Can you work these out from the model? Positions are in its coordinate system, mm. Face numbers are marked on the shaded views. A direction names the side the tool comes from. Give positions to 0.01 mm unless a question says otherwise; leave off trailing zeros. Loops run counter-clockwise (first coordinate to the right, second up) from the corner with the lowest first, then second, coordinate; pieces in that order, holes last. Notation, with made-up numbers: (36, -10.5) -> (79, -10.5) arc R23 ccw to (79, 11.5) -> close; hole circle Ø11 at (-10, -31.5). An arc over 180 degrees is marked (long way). One line per question, with ' | ' between items.
Autodesk Inventor part; units mm, degrees
ref_plane "YZ Plane" through (0, 0, 0) normal (1, 0, 0) x (0, 1, 0)
ref_plane "XZ Plane" through (0, 0, 0) normal (0, 1, 0) x (-1, 0, 0)
ref_plane "XY Plane" through (0, 0, 0) normal (0, 0, 1) x (1, 0, 0)
ref_plane "Work Plane1" through (0, 0, 0) normal (0, 0, 1) x (1, 0, 0)
ref_plane "Work Plane2" through (0, 0, 0) normal (0, 0, 1) x (1, 0, 0)
ref_plane "Work Plane3" through (0, 0, 0) normal (0, 0, 1) x (1, 0, 0)
sketch "Sketch1" plane through (0, 0, 0) normal (0, 0, 1) x (1, 0, 0)
  line L0 (232.95, -21.7) -> (142.052, -21.7)
  line L1 (142.052, -21.7) -> (142.052, 21.7)
  line L2 (142.052, 21.7) -> (232.95, 21.7)
  line L3 (232.95, 21.7) -> (232.95, -21.7)
  line L4 (148.402, -7.551111) -> (148.402, 7.551111)
  line L5 (226.6, 7.551111) -> (226.6, -7.551111)
  line L6 (205.085111, -9) -> (189.982889, -9)
  line L7 (188.534, 9) -> (206.534, 9)
  circle A0 centre (217.6, 0) radius 2.775
  circle A1 centre (217.6, 0) radius 5.315
  circle A2 centre (197.534, 0) radius 5.315
  circle A3 centre (177.468, 0) radius 5.315
  circle A4 centre (157.402, 0) radius 5.315
  circle A5 centre (217.6, 0) radius 2.775
  circle A6 centre (197.534, 0) radius 2.775
  circle A7 centre (177.468, 0) radius 2.775
  circle A8 centre (157.402, 0) radius 2.775
  line L8 (208.075, 9.906) -> (227.125, 9.906)
  line L9 (227.125, 9.906) -> (227.125, -9.906)
  line L10 (227.125, -9.906) -> (208.075, -9.906)
  line L11 (208.075, -9.906) -> (208.075, 9.906)
  line L12 (208.075, 9.906) -> (227.125, -9.906) construction
  line L13 (227.125, 9.906) -> (208.075, -9.906) construction
  line L14 (207.059, -9.906) -> (188.009, -9.906)
  line L15 (207.059, 9.906) -> (207.059, -9.906)
  line L16 (188.009, 9.906) -> (207.059, 9.906)
  line L17 (188.009, -9.906) -> (188.009, 9.906)
  line L18 (186.993, -9.906) -> (167.943, -9.906)
  line L19 (186.993, 9.906) -> (186.993, -9.906)
  line L20 (167.943, 9.906) -> (186.993, 9.906)
  line L21 (167.943, -9.906) -> (167.943, 9.906)
  line L22 (166.927, -9.906) -> (147.877, -9.906)
  line L23 (166.927, 9.906) -> (166.927, -9.906)
  line L24 (147.877, 9.906) -> (166.927, 9.906)
  line L25 (147.877, -9.906) -> (147.877, 9.906)
  point P0 (0, 0)
  dimension "d0" = 6.35
  dimension "d1" = 6.35
  dimension "d3" = 12.7
  dimension "d4" = 12.7
  dimension "d5" = 2.54
  dimension "d8" = 20.066
  dimension "d15" = 20.066
  dimension "d20" = 19.05
  dimension "d21" = 19.812
  dimension "d24" = 20.066
extrude "Extrusion1" add sketch "Sketch1" along normal blind 5 contours A1
sketch "Sketch3" plane through (0, 0, 0) normal (0, 0, 1) x (1, 0, 0)
  line L0 (225.6, -8) -> (209.6, -8)
  line L1 (225.6, 8) -> (225.6, -8)
  line L2 (209.6, 8) -> (225.6, 8)
  line L3 (209.6, -8) -> (209.6, 8)
  line L4 (210.616, -6.984) -> (224.584, -6.984)
  line L5 (224.584, -6.984) -> (224.584, 6.984)
  line L6 (224.584, 6.984) -> (210.616, 6.984)
  line L7 (210.616, 6.984) -> (210.616, -6.984)
  circle A0 centre (217.6, 0) radius 5.315
  circle A1 centre (217.6, 0) radius 2.775
  point P0 (0, 0)
  dimension "d40" = 1.016
sketch "Sketch3 outline for Extrusion3" plane through (0, 0, 0) normal (0, 0, 1) x (1, 0, 0)
  line L0 (210.616, -6.984) -> (224.584, -6.984)
  line L1 (210.616, 6.984) -> (210.616, -6.984)
  line L2 (224.584, -6.984) -> (224.584, 6.984)
  line L3 (224.584, 6.984) -> (210.616, 6.984)
  circle A0 centre (217.6, 0) radius 2.775
extrude "Extrusion3" add sketch "Sketch3 outline for Extrusion3" along normal blind 4 draft -15
pattern_linear "Rectangular Pattern1" count 4 spacing 20.066 along (-1, 0, 0) of "Extrusion3", "Extrusion1"
ref_plane "Work Plane4" through (0, 0, 0) normal (0, 0, 1) x (1, 0, 0)
sketch "Sketch4" plane through (0, 0, 0) normal (0, 0, 1) x (1, 0, 0)
  line L0 (-228.6, 12.7) -> (228.6, 12.7)
  line L1 (228.6, -12.7) -> (-228.6, -12.7)
  line L2 (228.6, 12.7) -> (228.6, -12.7)
  line L3 (146.336, 9) -> (146.336, -9)
  line L4 (228.6, 12.7) -> (146.336, 12.7)
  line L5 (146.336, 12.7) -> (146.336, -12.7)
  line L6 (146.336, -12.7) -> (228.6, -12.7)
  line L7 (228.6, -12.7) -> (228.6, 12.7)
  point P0 (0, 0)
extrude "Extrusion4" add sketch "Sketch4" against normal blind 4
properties part number "Bottom Holder"
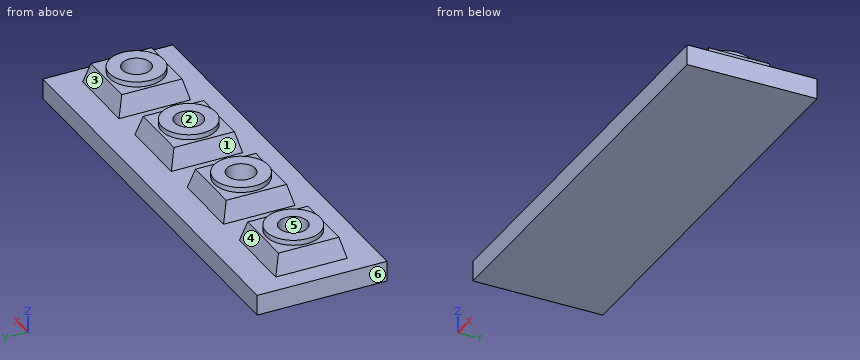
Q1. If we section it at A-A (x = 217.6): Write out the boundary of the cut face in (y, z) (3 decimals), plus the area to 3 significant figures.
Entries:
outline: (-12.7, -4) -> (12.7, -4) -> (12.7, 0) -> (6.984, 0) -> (5.912, 4) -> (5.315, 4) -> (5.315, 5) -> (2.775, 5) -> (2.775, 0) -> (-2.775, 0) -> (-2.775, 5) -> (-5.315, 5) -> (-5.315, 4) -> (-5.912, 4) -> (-6.984, 0) -> (-12.7, 0) -> close | area: 136 mm²
Q2. If I drill on probe 1 along Z at (x, y) = (215.5, 0.25); probe 2 along Y at (x, z) = (217.6, 2.7) (3 decimals); probe 3 along Y at (x, z) = (175.5, 1.5), over which ranges is the centre line in solid material (lowest first)? Write a range as from..to.
Entries:
probe 1: -4..0 | probe 2: -6.261..-2.775, 2.775..6.261 | probe 3: -6.58..-1.96, 1.96..6.58
Q3. If we section it at D-D (x = 168.5): Write out the boundary of the cut face in (y, z).
Entries:
outline: (-12.7, -4) -> (12.7, -4) -> (12.7, 0) -> (-12.7, 0) -> close
Q4. If we section it at B-B (x = 181): Write out the boundary of the cut face in (y, z), plus the area to 3 significant figures.
Entries:
outline: (-12.7, -4) -> (12.7, -4) -> (12.7, 0) -> (6.98, 0) -> (5.91, 4) -> (3.97, 4) -> (3.97, 5) -> (-3.97, 5) -> (-3.97, 4) -> (-5.91, 4) -> (-6.98, 0) -> (-12.7, 0) -> close | area: 161 mm²
Q5. For pin 1 Ø6 at (x, y) = (176, 1.5) entering from +Z; pin 2 Ø1.7 at (x, y) = (198, 0.5) entering from +Z; pin 3 Ø2 at (y, z) = (5.5, 2.5) entering from +X; pin 4 Ø1.5 at (x, z) = (158, 1) entering from -Y, each with a flat end and sliding along its axis, tell me the tip position at first contact or that it passes through.
Entries:
pin 1: z = 5 | pin 2: z = 0 | pin 3: x = 224.18 | pin 4: y = -6.92
Q6. If we section it at C-C (x = 156.5): Write out the boundary of the cut face in (y, z).
Entries:
outline: (-12.7, -4) -> (12.7, -4) -> (12.7, 0) -> (6.98, 0) -> (5.91, 4) -> (5.24, 4) -> (5.24, 5) -> (2.62, 5) -> (2.62, 0) -> (-2.62, 0) -> (-2.62, 5) -> (-5.24, 5) -> (-5.24, 4) -> (-5.91, 4) -> (-6.98, 0) -> (-12.7, 0) -> close
Q7. On a 3-axis mill with a long thin cutter (end or side, diameter ignored), from which of +Z, -Z, +X, -X, +Y, -Y can I reach the whole of each face in a straight line? I mean the marked faces 1, 2 and 3. Say none if no direction works.
Entries:
face 1: +Z, +Y, -Y | face 2: +Z | face 3: +Z, +X, -X, +Y
Q8. If we mould it in two halves opening along Y, with no side actions, what happens to the marked faces 4, 5 and 6? For each: pulls with the +Y half, pulls with the -Y half, needs draft (parallel to the pull), parting line crosses it, or undercut.
Entries:
face 4: pulls with the +Y half | face 5: undercut | face 6: needs draft
